Design review of the part built by this model. Coordinates are the model's own, in mm. Coordinates: 2 decimals unless noted, no trailing zeros. Write each loop counter-clockwise with the first axis right and the second up, starting at its lowest first coordinate (ties: lowest second). Pieces come first, ordered by that corner, then holes. Notation, with made-up numbers: M 28,-29.5 L 79,-29.5 A33 cw 79,5.5 Z; hole C 3.25,33 d5. An arc over 180 degrees is marked long. Return JSON: item names as keys, results as strings. Group by question number.
```python
from build123d import *

# Parameters (mm, degrees)
SKETCH_R  = 3
PAD_DEPTH = 10


with BuildPart() as part:
    # Sketch → Pad (new body)
    with BuildSketch(Plane.XY):
        with BuildLine():
            Line((-31, 14), (0, 14))
            ThreePointArc((8.85963, -10.840063), (13.186373, 4.703144), (0, 14))
            ThreePointArc((8.85963, -10.840063), (-8.278867, -33.56864), (-13.013103, -61.638256))
            ThreePointArc((-18, -67), (-14.338803, -65.405237), (-13.013103, -61.638256))
            Line((-18, -67), (-31, -67))
            ThreePointArc((-36, -62), (-34.535534, -65.535534), (-31, -67))
            Line((-36, -62), (-36, 9))
            ThreePointArc((-31, 14), (-34.535534, 12.535534), (-36, 9))
        make_face()
        with Locations((-27, 0)):
            Circle(SKETCH_R, mode=Mode.SUBTRACT)
        Circle(SKETCH_R, mode=Mode.SUBTRACT)
    extrude(amount=PAD_DEPTH)


solid = part.part
```
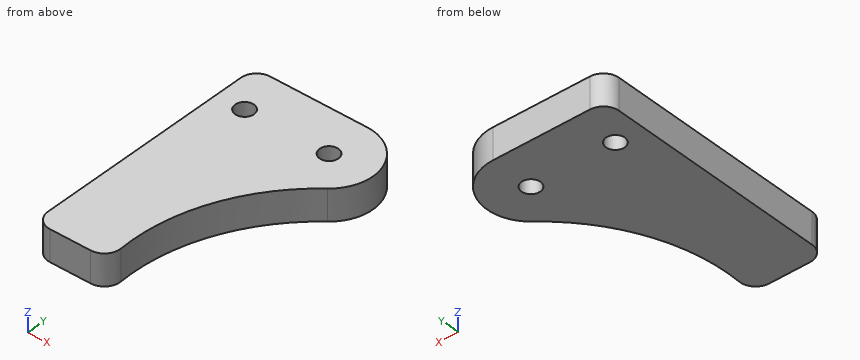
Item 1: For line 1 (Y direction, x = -27, z = 4.25); line 2 (X direction, y = -2, z = 8.5); line 3 (X direction, y = -39, z = 1), list the stretches that pass through material, from the lowest coordinate up.
Item 2: For pin 1 (4 mm diameter, centred on x = -2, y = -28, fed in from -Z); pin 2 (3 mm diameter, centred on y = -7.5, z = 5.5, fed in from +X); pin 3 (2 mm diameter, centred on x = -7, z = 5, fed in from -Y), all flat-tipped, find the tip position at first contact; note any pin that passes through.
Item 3: Add section A-A (x = -27). Write out the cut boundary in (y, z), plus the area to 3 significant figures.
Item 4: Add section D-D (x = -5). Write out the cut boundary in (y, z), plus the area to 3 significant figures.
Item 5: Add section C-C (z = 9). Write out the cut boundary in (x, y), plus the area to 3 significant figures.
Item 6: Add section B-B (y = 0). Write out the cut boundary in (x, z).
Geometry check:
{
 "1": {"line 1": "-67 to -3, 3 to 14", "line 2": "-36 to -29.24, -24.76 to -2.24, 2.24 to 13.86", "line 3": "-36 to -10.31"},
 "2": {"pin 1": "through", "pin 2": "x = 12.65", "pin 3": "y = -32.93"},
 "3": {"outline": "M -67,0 L -3,0 L -3,10 L -67,10 Z; M 3,0 L 14,0 L 14,10 L 3,10 Z", "area": "750 mm^2"},
 "4": {"outline": "M -27.07,0 L 14,0 L 14,10 L -27.07,10 Z", "area": "411 mm^2"},
 "5": {"outline": "M -36,-62 A5 ccw -31,-67 L -18,-67 A5 ccw -13.01,-61.64 A60 cw 8.86,-10.84 A14 ccw 0,14 L -31,14 A5 ccw -36,9 Z; hole C -27,0 d6; hole C 0,0 d6", "area": "2,700 mm^2"},
 "6": {"outline": "M -36,0 L -30,0 L -30,10 L -36,10 Z; M -24,0 L -3,0 L -3,10 L -24,10 Z; M 3,0 L 14,0 L 14,10 L 3,10 Z"}
}
